Build history of the part. All positions in model axes, mm. Face numbers are marked on the shaded views. A direction names the side the tool comes from. Round coordinates to 2 decimals unless told otherwise and drop trailing zeros. Order: outer loops, then holes, each group sorted by start corner. A loop starts at its lowest first (then second) coordinate and runs counter-clockwise, first axis right, second up. Notation, with made-up numbers: M 78,1 L 127,1 A11 ccw 127,21 Z; hole C -5,5.5 d6. An arc over 180 degrees is marked long. One line per item, written item: value. Start each with the question number.
Item 1: Band-saw the part on A-A, the plane z = 3.5. Write the cut outline in (x, y), then the cut area to 3 significant figures.
Item 2: Pin check, flat tips, straight feed: pin 1 (6 mm diameter, centred on y = 2.5, z = -4, fed in from +X); pin 2 (3.5 mm diameter, centred on x = 16, y = 1.5, fed in from -Z); pin 3 (2 mm diameter, centred on x = -17, z = 7.5, fed in from +Y); pin 4 (2.5 mm diameter, centred on x = -7, z = -14, fed in from -Y). Stop position of each tip, or through.
Item 3: Two-plate mould, pull along X, no slides. Class the marked faces 1, 2 and 3: +X half, -X half, draft (parallel to the pull), parting line (faces both ways), or undercut.
Item 4: Band-saw the part on B-B, the plane x = -16.5. Write the cut outline in (y, z), then the cut area to 3 significant figures.
Item 5: Tool access for the marked faces 4, 5, 6 and 7: list every direction of +Z, -Z, +X, -X, +Y, -Y with a clear straight run to the whole face (end or side of a thin tool).
Item 6: Band-saw the part on C-C, the plane z = -14. Write the cut outline in (x, y) (3 decimals), then the cut area to 3 significant figures.
Item 7: Probe L1, parallel to Z at x = 16.5, y = 1.7; L2, parallel to Z at x = -7, y = 7.75; L3, parallel to X at y = 2.5, z = -14. List the from-to ranges inside material, lowest first.
Item 8: Band-saw the part on D-D, the plane x = -8. Write the cut outline in (y, z), then the cut area to 3 significant figures.
```python
from build123d import *

# Parameters (mm, degrees)
F1_ANGLE = 180
F2_W     = 9
F2_H     = 22
F3_DEPTH = 3
F4_D     = 3.3
F8_DEPTH = 30


with BuildPart() as f1:
    # F0 (on Front) → F1 (revolve)
    with BuildSketch(Plane.XZ):
        Polygon((-12, 21), (-11, 21), (-11, 22), (-14, 22), (-14, -21), (0, -21), (0, -1), (-11, -1), (-11, 0), (-12, 0), (-12, 7), (-11, 7), (-11, 14), (-12, 14), align=None)
    revolve(axis=Axis((0, 0, -11), (0, 0, -1)), revolution_arc=F1_ANGLE)

    # F2 (on face) → F3 (join)
    with BuildSketch(Plane.XZ):
        with Locations((-16.5, 11)):
            Rectangle(F2_W, F2_H)
        with Locations((16.5, 11)):
            Rectangle(F2_W, F2_H)
    extrude(amount=-F3_DEPTH)

    # F4 (through all)
    with Locations(Plane.XZ):
        with Locations((-16.5, 18.5), (-16.5, 3.5), (-7, -14), (16.5, 18.5), (16.5, 3.5)):
            Hole(F4_D / 2)

    # F7 (on offset) → F8 (cut)
    with BuildSketch(Plane(origin=(4.4739377588, 0, 6.5075458311), x_dir=(0.8240419242, 0, -0.5665288229), z_dir=(-0.5665288229, 0, -0.8240419242))):
        Polygon((16.5365869388, -5), (21.5365869388, 0), (11.5365869388, 0), align=None)
    extrude(amount=F8_DEPTH, mode=Mode.SUBTRACT)


solid = f1.part
```
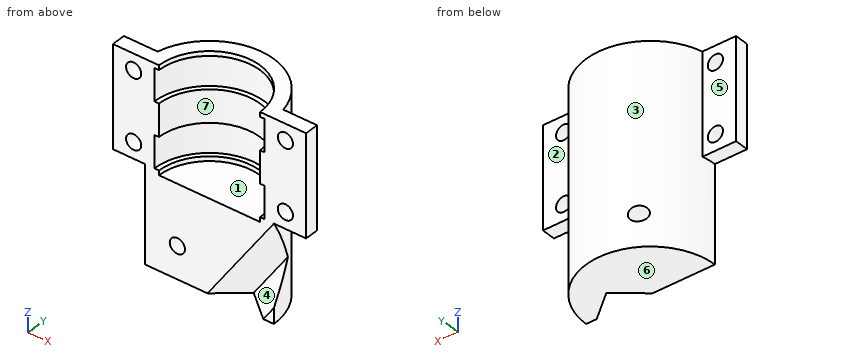
Output:
1. outline: M -21,0 L -18.15,0 L -18.15,3 L -21,3 Z; M -14.85,0 L -12,0 A12 cw 12,0 L 14.85,0 L 14.85,3 L 13.67,3 A14 ccw -13.67,3 L -14.85,3 Z; M 18.15,0 L 21,0 L 21,3 L 18.15,3 Z
1. area: 105 mm²
2. pin 1: stops at x = 13.98
2. pin 2: stops at z = 0
2. pin 3: stops at y = 3
2. pin 4: passes through
3. face 1: undercut
3. face 2: draft
3. face 3: parting line
4. outline: M 0,0 L 3,0 L 3,1.85 L 0,1.85 Z; M 0,5.15 L 3,5.15 L 3,16.85 L 0,16.85 Z; M 0,20.15 L 3,20.15 L 3,22 L 0,22 Z
4. area: 46.2 mm²
5. face 4: -Y
5. face 5: +Z, -Z, -X, +Y
5. face 6: -Z, +X, -X, +Y, -Y
5. face 7: +Z, -Y
6. outline: M -14,0 L -8.65,0 L -8.65,11.008 A14 ccw Z; M -5.35,0 L 4.375,0 L 10.443,5 L 13.824,2.214 A14 ccw -5.35,12.937 Z
6. area: 240 mm²
7. L1: z = 0 to 1.85, 5.15 to 16.85, 20.15 to 22
7. L2: z = -21 to -15.65, -12.35 to -1
7. L3: x = -13.77 to -8.65, -5.35 to 7.41, 13.48 to 13.77
8. outline: M 0,-21 L 11.49,-21 L 11.49,-15.31 L 0,-15.31 Z; M 0,-12.69 L 11.49,-12.69 L 11.49,22 L 7.55,22 L 7.55,21 L 8.94,21 L 8.94,14 L 7.55,14 L 7.55,7 L 8.94,7 L 8.94,0 L 7.55,0 L 7.55,-1 L 0,-1 Z
8. area: 271 mm²
